The listing builds one solid part. Answer for the finished solid, in the listing's coordinates (mm). A direction names the side the tool comes from. Coordinates: 2 decimals unless noted, no trailing zeros. Order: outer loops, then holes, each group sorted by start corner. A loop starts at its lowest first (then second) coordinate and runs counter-clockwise, first axis right, second up. Notation, with made-up numbers: M -5.5,59.5 L 8.5,59.5 A13 ccw 8.5,79.5 Z; hole C 46.25,24 d9. An arc over 180 degrees is marked long. One line per item, written item: value. Start each with the question number.
Q1. The part is cut by section D-D on x = -52.5. Give the vertices of the cut face in (y, z), then the cut area to 3 significant figures.
Q2. Each of these flat-tipped pins is pushed along its axis until it touches: pin 1 Ø2 at (x, z) = (-15, 56) entering from +Y; pin 2 Ø1.5 at (x, y) = (-57.5, -39) entering from -Z; pin 3 Ø15 at (x, y) = (-29, -38.5) entering from -Z; pin 4 Ø5 at (x, y) = (-49, -43) entering from +Z. Where does it stop, or does it pass through?
Q3. Determine the mould class of faces 1 (the flat face through (-35, -35, 67.38)), 2 (the flat face through (-54, -60.8, -12)), 3 (the flat face through (-35, -10, 20)) for opening direction Z: pulls with the +Z half, pulls with the -Z half, needs draft (parallel to the pull), parting line crosses it, or undercut.
Q4. The part is cut by section A-A on z = 40. Give the vertices of the cut face in (x, y), then the cut area to 3 significant figures.
Q5. The part is cut by section C-C on y = -29. Give the vertices of the cut face in (x, z).
Q6. Straight lines are drawn through the part: line 1 along Y through (x, z) = (-4, 45); line 2 along Z through (x, y) = (-21, -56); line 3 along Z through (x, y) = (-49.5, -44.5). For each, find the intervals that lie inside material, in ascending order. Write a range as [from, to].
Q7. For faces 4 (the flat face through (-35, -5, -35.396)), 5 (the flat face through (-35, -35, 37.38)), 6 (the flat face through (-64.277, -35, 52)), 7 (the flat face through (-4.277, -35, 52)), determine the directions among +Z, -Z, +X, -X, +Y, -Y from which every point of the face is accessible in a straight line to the end or side of a thin tool.
Q8. The part is cut by section B-B on x = -22. Give the vertices of the cut face in (y, z).
```python
from build123d import *

# Parameters (mm, degrees)
F0_W     = 69.50178
F0_H     = 109.138066
F1_DEPTH = 10
F2_W     = 60
F2_H     = 30
F4_DEPTH = 50.8
F5_DEPTH = 50.8


with BuildPart() as f1:
    # F0 (on Front) → F1 (new body)
    with BuildSketch(Plane.XZ):
        with Locations((-34.75089, 19.172902)):
            Rectangle(F0_W, F0_H)
    extrude(amount=F1_DEPTH)

    # F2 (on face) → F4 (join)
    with BuildSketch(Plane.XZ.offset(10)):
        with Locations((-34.276575, 52.379627)):
            Rectangle(F2_W, F2_H)
    extrude(amount=F4_DEPTH)

    # F3 (on face) → F5 (join)
    with BuildSketch(Plane.XZ.offset(10)):
        with BuildLine():
            ThreePointArc((-69.50178, -13.655613), (-53.107139, -27.798143), (-38.17735, -12.117047))
            ThreePointArc((-38.17735, -12.117047), (-53.107139, 3.564049), (-69.50178, -10.578481))
            Line((-69.50178, -10.578481), (-69.50178, -13.655613))
        make_face()
    extrude(amount=F5_DEPTH)


solid = f1.part
```
Output:
1. outline: M -60.8,-27.76 L -10,-27.76 L -10,-35.4 L 0,-35.4 L 0,73.74 L -10,73.74 L -10,67.38 L -60.8,67.38 L -60.8,37.38 L -10,37.38 L -10,3.52 L -60.8,3.52 Z
1. area: 4,200 mm^2
2. pin 1: stops at y = 0
2. pin 2: stops at z = -27.55
2. pin 3: stops at z = 37.38
2. pin 4: stops at z = 67.38
3. face 1: pulls with the +Z half
3. face 2: needs draft
3. face 3: undercut
4. outline: M -69.5,-10 L -64.28,-10 L -64.28,-60.8 L -4.28,-60.8 L -4.28,-10 L 0,-10 L 0,0 L -69.5,0 Z
4. area: 3,740 mm^2
5. outline: M -69.5,-13.66 A15.7 ccw long -69.5,-10.58 Z; M -64.28,37.38 L -4.28,37.38 L -4.28,67.38 L -64.28,67.38 Z
6. line 1: y = [-10, 0]
6. line 2: z = [37.38, 67.38]
6. line 3: z = [-27.19, 2.96], [37.38, 67.38]
7. face 4: -Z, +X, -X, +Y, -Y
7. face 5: +X, -X, -Y
7. face 6: +Z, -X, -Y
7. face 7: +Z, -Z, +X, -Y
8. outline: M -60.8,37.38 L -10,37.38 L -10,-35.4 L 0,-35.4 L 0,73.74 L -10,73.74 L -10,67.38 L -60.8,67.38 Z
